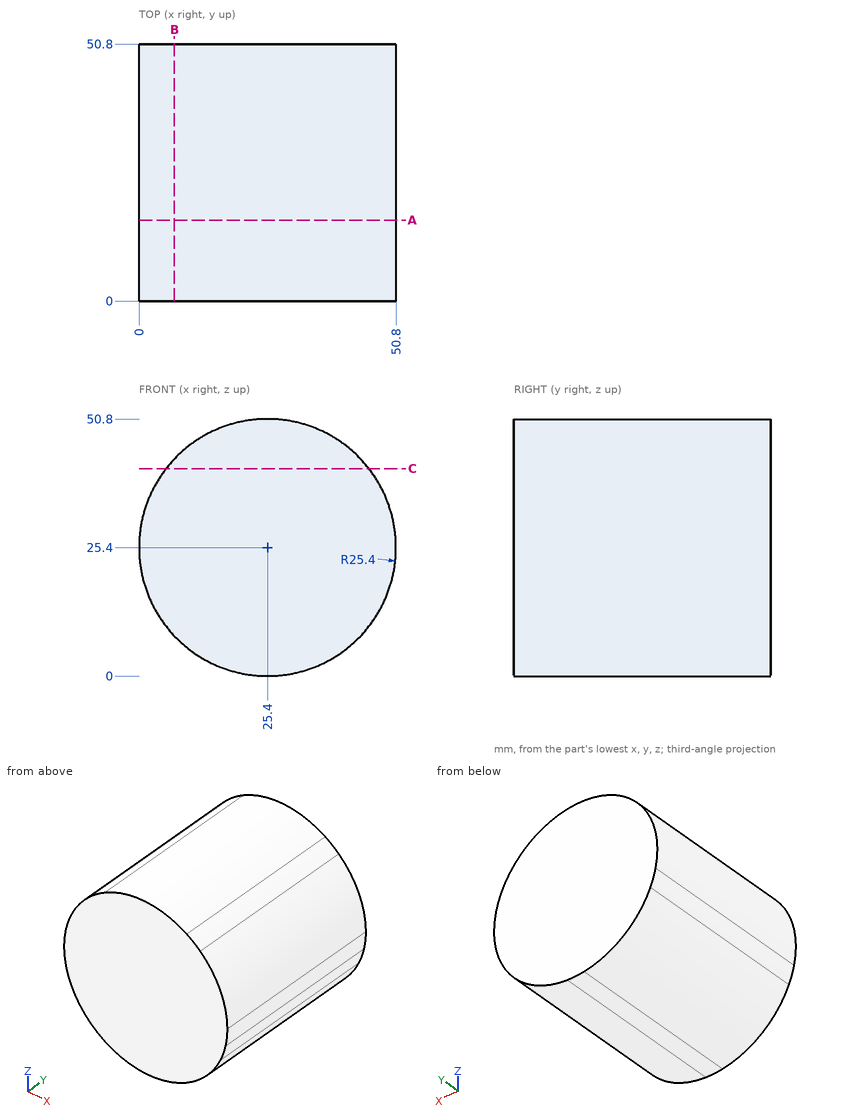
Geometry: see drawing. Coordinates: mm, zero at the bounding-box minimum. Round coordinates to 2 decimals unless told otherwise and drop trailing zeros. Loops run counter-clockwise (first coordinate to the right, second up) from the corner with the lowest first, then second, coordinate; pieces in that order, holes last. Notation, with made-up numbers: (-1.75, 80.5) - (25.25, 80.5) arc R18 cw to (25.25, 98.5) - close; hole circle Ø4 at (17.5, 79). An arc over 180 degrees is marked (long way). One line per item, written item: value. Start each with the question number.
(1) Section C-C, the plane z = 41. Return loops of the section in (x, y), plus the area to 3 significant figures.
(2) Ray query, line 1 (Z direction, x = 26, y = 36); line 2 (X direction, y = 33, z = 25); line 3 (X direction, y = 15, z = 20). Return the intervals inside material, ascending. Write a range as [from, to].
(3) Contact query for flat-ended pins moving along their axis: P1, Ø3, axis at x = 8, y = 16.5, coming from the +Z side; P2, Ø12, axis at x = 14, y = 30.5, coming from the +Z side; P3, Ø2, axis at x = 23.5, y = 21.5, coming from the -Z side. Output: stop coordinate, or through.
(4) Section B-B, the plane x = 7. Return loops of the section in (y, z).
(5) Section A-A, the plane y = 16. Return loops of the section in (x, z), plus the area to 3 significant figures.
Results below:
1. outline: (5.36, 0) - (45.44, 0) - (45.44, 50.8) - (5.36, 50.8) - close
1. area: 2,040 mm^2
2. line 1: [0.01, 50.79]
2. line 2: [0, 50.8]
2. line 3: [0.58, 50.22]
3. P1: z = 45.21
3. P2: z = 50.22
3. P3: z = 0.02
4. outline: (0, 7.89) - (50.8, 7.89) - (50.8, 42.91) - (0, 42.91) - close
5. outline: circle Ø50.8 at (25.4, 25.4)
5. area: 2,030 mm^2
